Input: part model. Units: mm. Frame: model coordinates. Face numbers are marked on the shaded views. A direction names the side the tool comes from. Give positions to 0.01 mm unless a question says otherwise; leave off trailing zeros. Order: outer loops, then holes, each group sorted by start corner. A loop starts at its lowest first (then second) coordinate and runs counter-clockwise, first axis right, second up. Notation, with made-up numbers: M 61.25,57 L 72.25,57 A37 ccw 72.25,96 Z; hole C 74,22.5 d9. An arc over 180 degrees is marked long. Use a Markdown table: item, result.
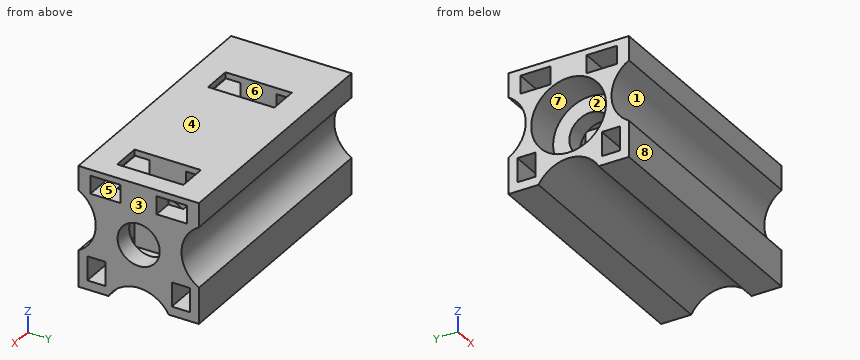
from build123d import *

# Parameters (mm, degrees)
SKETCH_R        = 1.75
PAD_DEPTH       = 21
SKETCH002_W     = 5.5
SKETCH002_H     = 2.4
POCKET_DEPTH    = 8
SKETCH003_R     = 3.1
POCKET001_DEPTH = 3
SKETCH007_W     = 1.5
SKETCH007_H     = 2
SKETCH007_W_2   = 2.5
SKETCH007_H_2   = 1.5
POCKET002_DEPTH = 21.001


with BuildPart() as part:
    # Sketch → Pad (new body)
    with BuildSketch(Plane.YZ):
        with BuildLine():
            Line((-5, 8), (-5, 10))
            Line((-5, 10), (5, 10))
            Line((5, 10), (5, 8))
            ThreePointArc((5, 8), (3.556624, 5.5), (5, 3))
            Line((5, 3), (5, 0))
            Line((5, 0), (2.5, 0))
            ThreePointArc((2.5, 0), (0, 1.443376), (-2.5, 0))
            Line((-2.5, 0), (-5, 0))
            Line((-5, 0), (-5, 3))
            ThreePointArc((-5, 3), (-3.556624, 5.5), (-5, 8))
        make_face()
        with Locations((0, 5)):
            Circle(SKETCH_R, mode=Mode.SUBTRACT)
    extrude(amount=PAD_DEPTH)

    # Sketch002 → Pocket (cut)
    with BuildSketch(Plane(origin=(0, 0, 10), x_dir=(0, -1, 0), z_dir=(0, 0, 1))):
        with Locations((0, 5.7)):
            Rectangle(SKETCH002_W, SKETCH002_H)
        with Locations((0, 18.2)):
            Rectangle(SKETCH002_W, SKETCH002_H)
    extrude(amount=-POCKET_DEPTH, mode=Mode.SUBTRACT)

    # Sketch003 (on Face4 of Pocket) → Pocket001 (cut)
    with BuildSketch(Plane(origin=(0, 0, 0), x_dir=(0, 1, 0), z_dir=(-1, 0, 0))):
        with Locations((0, -5)):
            Circle(SKETCH003_R)
    extrude(amount=-POCKET001_DEPTH, mode=Mode.SUBTRACT)

    # Sketch007 (on Face4 of Pocket001) → Pocket002 (cut, through all)
    with BuildSketch(Plane(origin=(0, 0, 0), x_dir=(0, 1, 0), z_dir=(-1, 0, 0))):
        with Locations((-3.5, -1.75)):
            Rectangle(SKETCH007_W, SKETCH007_H)
        with Locations((3.5, -1.75)):
            Rectangle(SKETCH007_W, SKETCH007_H)
        with Locations((-2.75, -8.75)):
            Rectangle(SKETCH007_W_2, SKETCH007_H_2)
        with Locations((2.75, -8.75)):
            Rectangle(SKETCH007_W_2, SKETCH007_H_2)
    extrude(amount=-POCKET002_DEPTH, mode=Mode.SUBTRACT)


solid = part.part
1) Cut plane C-C on x = 14.5. Return loops of the section in (y, z), and give its area (3 significant figures).
Response values:
| item | result |
|---|---|
| outline | M -5,0 L -2.5,0 A2.89 cw 2.5,0 L 5,0 L 5,3 A2.89 cw 5,8 L 5,10 L -5,10 L -5,8 A2.89 cw -5,3 Z; hole M -4.25,0.75 L -2.75,0.75 L -2.75,2.75 L -4.25,2.75 Z; hole M -4,8 L -1.5,8 L -1.5,9.5 L -4,9.5 Z; hole C 0,5 d3.5; hole M 1.5,8 L 4,8 L 4,9.5 L 1.5,9.5 Z; hole M 2.75,0.75 L 4.25,0.75 L 4.25,2.75 L 2.75,2.75 Z |
| area | 61.5 mm² |
2) Reachability of the marked faces 5, 6, 7 and 8 from +Z, -Z, +X, -X, +Y, -Y: full face, straight path, thin tool, end or side. Return the list, or none.
Response values:
| item | result |
|---|---|
| face 5 | +X, -X |
| face 6 | +Z |
| face 7 | -X |
| face 8 | +Z, -Z, +X, -X, -Y |
3) Mould query, pull axis Z, two halves, no side actions, for the marked faces 1, 2, 3 and 4. Classes: released by +Z, released by -Z, zero draft, split by the parting line, or undercut.
Response values:
| item | result |
|---|---|
| face 1 | undercut |
| face 2 | undercut |
| face 3 | zero draft |
| face 4 | released by +Z |
4) Material intervals for line 1 (X direction, y = 2.5, z = 3); line 2 (Y direction, x = 9, z = 9.25); line 3 (Y direction, x = 2.75, z = 1.75), sorted ascending. Write a range as from..to.
Response values:
| item | result |
|---|---|
| line 1 | x = 0..4.5, 6.9..17, 19.4..21 |
| line 2 | y = -5..-4, -1.5..1.5, 4..5 |
| line 3 | y = -5..-4.25, -2.75..2.75, 4.25..5 |
5) First-contact query: pin 1 Ø4 at (y, z) = (0, 5) entering from -X; pin 2 Ø1.9 at (x, z) = (18, 6) entering from -Y; pin 3 Ø3 at (x, y) = (3, 0.5) entering from -Z. Flat tips, straight axial feed; report the tip coordinate or a pass-through.
Response values:
| item | result |
|---|---|
| pin 1 | stops at x = 3 |
| pin 2 | stops at y = -3.95 |
| pin 3 | stops at z = 0.64 |
6) Cut plane B-B on z = 8.75. Return loops of the section in (x, y).
Response values:
| item | result |
|---|---|
| outline | M 0,-5 L 21,-5 L 21,-4 L 0,-4 Z; M 0,-1.5 L 4.5,-1.5 L 4.5,1.5 L 0,1.5 Z; M 0,4 L 21,4 L 21,5 L 0,5 Z; M 6.9,-1.5 L 17,-1.5 L 17,1.5 L 6.9,1.5 Z; M 19.4,-1.5 L 21,-1.5 L 21,1.5 L 19.4,1.5 Z |
7) Cut plane A-A on y = 0. Return loops of the section in (x, z).
Response values:
| item | result |
|---|---|
| outline | M 0,1.44 L 21,1.44 L 21,3.25 L 19.4,3.25 L 19.4,2 L 17,2 L 17,3.25 L 6.9,3.25 L 6.9,2 L 4.5,2 L 4.5,3.25 L 3,3.25 L 3,1.9 L 0,1.9 Z; M 0,8.1 L 3,8.1 L 3,6.75 L 4.5,6.75 L 4.5,10 L 0,10 Z; M 6.9,6.75 L 17,6.75 L 17,10 L 6.9,10 Z; M 19.4,6.75 L 21,6.75 L 21,10 L 19.4,10 Z |
